Build history of the part. All positions in model axes, mm. Face numbers are marked on the shaded views. A direction names the side the tool comes from. Round coordinates to 2 decimals unless told otherwise and drop trailing zeros. Write each loop counter-clockwise with the first axis right and the second up, starting at its lowest first coordinate (ties: lowest second). Pieces come first, ordered by that corner, then holes.
Item 1: Band-saw the part on A-A, the plane z = 12.5. Write the cut outline in (x, y), then the cut area to 3 significant figures.
Item 2: Wall check: probe 1 along Y at (x, z) = (-3, 20.5); probe 2 along X at (y, z) = (-4, 12.5); probe 3 along Z at (x, y) = (8, -19.75). Give the ranges that are in metal, low to high.
Item 3: Band-saw the part on D-D, the plane y = -13.5. Write the cut outline in (x, z), then the cut area to 3 significant figures.
Item 4: Band-saw the part on B-B, the plane x = -21.5. Write the cut outline in (y, z).
Item 5: Band-saw the part on C-C, the plane y = -23.25. Write the cut outline in (x, z), then the cut area to 3 significant figures.
Item 6: Drop flat-ended pins along their axis: pin 1 Ø4.5 at (x, y) = (-6.5, -9) entering from -Z; pin 2 Ø24 at (x, z) = (-5, 9.5) entering from +Y; pin 3 Ø1.3 at (x, y) = (4, -2.5) entering from -Z. Give the stop position or say it passes through.
Item 7: Mould opens along Y. For the marked faces 3, 4 and 5 say: +Y half, -Y half, draft (parallel to the pull), parting line (faces both ways), or undercut.
Item 8: 3-axis set-ups, long thin cutter, end or side, ignore diameter. For the marked faces 1 and 2: which of +Z, -Z, +X, -X, +Y, -Y reach the whole face in a straight line?
```python
from build123d import *

# Parameters (mm, degrees)
F0_W     = 50.8
F0_H     = 50.8
F1_DEPTH = 25.4
F2_W     = 30.48
F2_H     = 45.72
F3_DEPTH = 25.401
F4_W     = 15.741314
F4_H     = 47.608288
F5_DEPTH = 50.801


with BuildPart() as f1:
    # F0 (on Front) → F1 (new body)
    with BuildSketch(Plane.XZ):
        Rectangle(F0_W, F0_H)
    extrude(amount=F1_DEPTH)

    # F2 (on face) → F3 (cut, through all)
    with BuildSketch(Plane.XZ.offset(25.4)):
        with Locations((0, -2.54)):
            Rectangle(F2_W, F2_H)
    extrude(amount=-F3_DEPTH, mode=Mode.SUBTRACT)

    # F4 (on face) → F5 (cut, through all)
    with BuildSketch(Plane.YZ.offset(25.4)):
        with Locations((-12.098421, -1.595856)):
            Rectangle(F4_W, F4_H)
    extrude(amount=-F5_DEPTH, mode=Mode.SUBTRACT)


solid = f1.part
```
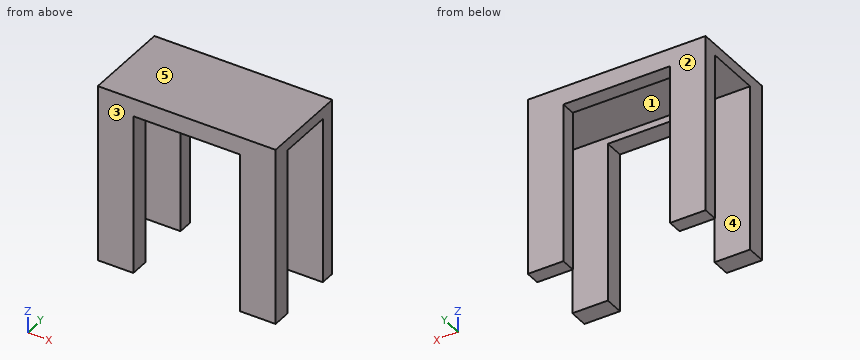
Results:
1. outline: (-25.4, -25.4) - (-15.24, -25.4) - (-15.24, -19.97) - (-25.4, -19.97) - close; (-25.4, -4.23) - (-15.24, -4.23) - (-15.24, 0) - (-25.4, 0) - close; (15.24, -25.4) - (25.4, -25.4) - (25.4, -19.97) - (15.24, -19.97) - close; (15.24, -4.23) - (25.4, -4.23) - (25.4, 0) - (15.24, 0) - close
1. area: 196 mm2
2. probe 1: y = -25.4 to -19.97, -4.23 to 0
2. probe 2: x = -25.4 to -15.24, 15.24 to 25.4
2. probe 3: z = 22.21 to 25.4
3. outline: (-25.4, 22.21) - (25.4, 22.21) - (25.4, 25.4) - (-25.4, 25.4) - close
3. area: 162 mm2
4. outline: (-25.4, -25.4) - (-19.97, -25.4) - (-19.97, 22.21) - (-4.23, 22.21) - (-4.23, -25.4) - (0, -25.4) - (0, 25.4) - (-25.4, 25.4) - close
5. outline: (-25.4, -25.4) - (-15.24, -25.4) - (-15.24, 20.32) - (15.24, 20.32) - (15.24, -25.4) - (25.4, -25.4) - (25.4, 25.4) - (-25.4, 25.4) - close
5. area: 1,190 mm2
6. pin 1: stops at z = 22.21
6. pin 2: stops at y = 0
6. pin 3: stops at z = 20.32
7. face 3: -Y half
7. face 4: undercut
7. face 5: draft
8. face 1: -Z, +X, -X
8. face 2: +Z, -Z, +X, -X, +Y
